The figure shows three views and two pictorial views of one solid part (mm, origin at its lowest corner). Answer the questions. Give positions to 0.01 mm unless a question says otherwise; leave off trailing zeros. Loops run counter-clockwise (first coordinate to the right, second up) from the corner with the lowest first, then second, coordinate; pieces in that order, holes last. Notation, with made-up numbers: M -17.75,-5 L 35.25,-5 A10 cw 35.25,8 Z; hole C -11,48 d11. An arc over 180 degrees is marked long. One line per item, written item: value. Start each with the question number.
Q1. A cutting plane is placed at D-D, the plane x = 148. Determine the outline of the cut face in (y, z).
Q2. Flat-ended cylindrical pins translate along their axes: pin 1 (2.5 mm diameter, centred on y = 104, z = 2, fed in from -X); pin 2 (2.5 mm diameter, centred on x = 104, z = 1.5, fed in from +Y); pin 3 (2.5 mm diameter, centred on x = 143, z = 2.5, fed in from +Y); pin 4 (3 mm diameter, centred on x = 113.5, z = 1.5, fed in from -Y). Find the tip coordinate at first contact, or state that the pin passes through.
Q3. A cutting plane is placed at C-C, the plane x = 107.5. Determine the outline of the cut face in (y, z), and give its area (3 significant figures).
Q4. A cutting plane is placed at B-B, the plane z = 3.35. Determine the outline of the cut face in (x, y), and give its area (3 significant figures).
Q5. A cutting plane is placed at A-A, the plane y = 68.5. Determine the outline of the cut face in (x, z), and give its area (3 significant figures).
Q6. Consider L1, parallel to X at y = 72, z = 0.95; L2, parallel to X at y = 78, z = 0.25; L3, parallel to X at y = 80.5, z = 2.75. Determine where each line is inside the solid, lowest interval first.
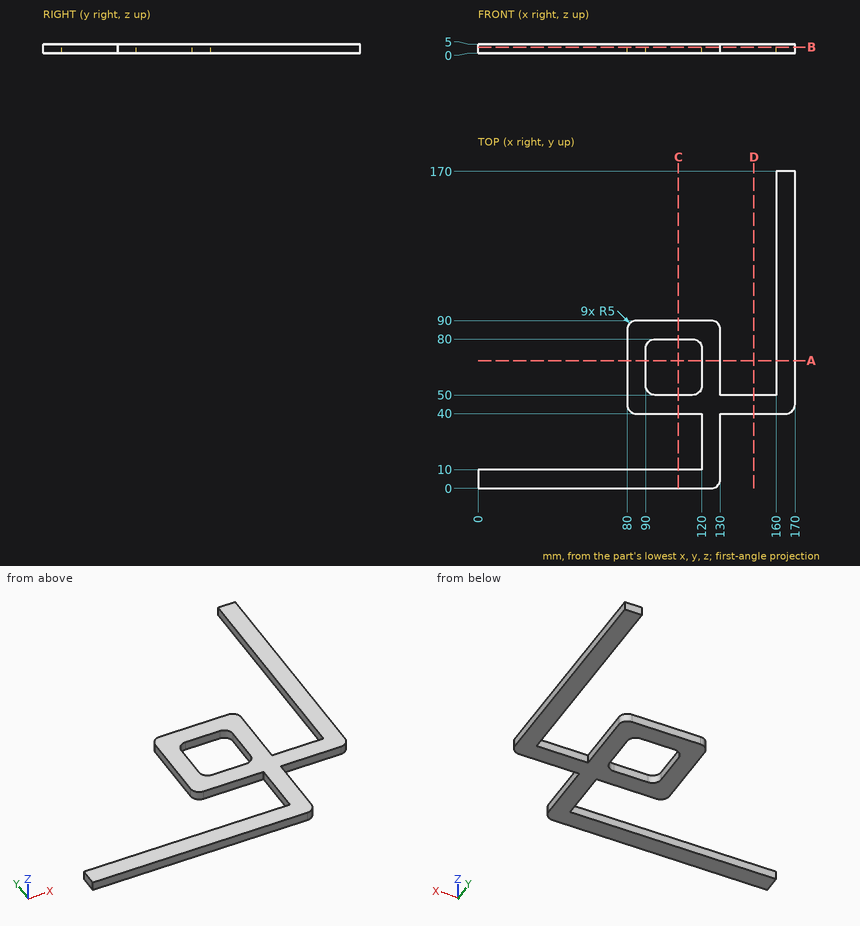
Answer block:
1. outline: M 40,0 L 50,0 L 50,5 L 40,5 Z
2. pin 1: x = 160
2. pin 2: y = 90
2. pin 3: y = 50
2. pin 4: y = 0
3. outline: M 0,0 L 10,0 L 10,5 L 0,5 Z; M 40,0 L 50,0 L 50,5 L 40,5 Z; M 80,0 L 90,0 L 90,5 L 80,5 Z
3. area: 150 mm^2
4. outline: M 0,0 L 125,0 A5 ccw 130,5 L 130,40 L 165,40 A5 ccw 170,45 L 170,170 L 160,170 L 160,50 L 130,50 L 130,85 A5 ccw 125,90 L 85,90 A5 ccw 80,85 L 80,45 A5 ccw 85,40 L 120,40 L 120,10 L 0,10 Z; hole M 90,55 A5 ccw 95,50 L 115,50 A5 ccw 120,55 L 120,75 A5 ccw 115,80 L 95,80 A5 ccw 90,75 Z
4. area: 4,790 mm^2
5. outline: M 80,0 L 90,0 L 90,5 L 80,5 Z; M 120,0 L 130,0 L 130,5 L 120,5 Z; M 160,0 L 170,0 L 170,5 L 160,5 Z
5. area: 150 mm^2
6. L1: 80 to 90, 120 to 130, 160 to 170
6. L2: 80 to 91, 119 to 130, 160 to 170
6. L3: 80 to 130, 160 to 170
